The listing builds one solid part. Answer for the finished solid, in the listing's coordinates (mm). Face numbers are marked on the shaded views. A direction names the side the tool comes from. Coordinates: 2 decimals unless noted, no trailing zeros. Order: outer loops, then holes, each group sorted by start corner. A loop starts at its lowest first (then second) coordinate and runs counter-clockwise, first axis right, second up. Notation, with made-up numbers: (66.25, 51) -> (108.25, 51) arc R18 ccw to (108.25, 84) -> close; hole circle Ø10 at (-6, 8.25). An arc over 180 degrees is marked (long way). Return JSON: item names as keys, results as strings.
from build123d import *

# Parameters (mm, degrees)
SKETCH_1_W          = 40
SKETCH_1_H          = 30
EXTRUDE_1_DEPTH     = 5
SKETCH_2_R          = 1.5
CUT_EXTRUDE_1_DEPTH = 10
SKETCH_3_W          = 20
SKETCH_3_H          = 30
CUT_EXTRUDE_2_DEPTH = 1


with BuildPart() as part:
    # 草图1 → 凸台-拉伸1 (new body)
    with BuildSketch(Plane.XY):
        Rectangle(SKETCH_1_W, SKETCH_1_H)
    extrude(amount=EXTRUDE_1_DEPTH)

    # 草图2 → 切除-拉伸1 (cut)
    with BuildSketch(Plane(origin=(0, 0, 0), x_dir=(-1, 0, 0), z_dir=(0, 0, -1))):
        with Locations((14, 10)):
            Circle(SKETCH_2_R)
        with Locations((-14, 10)):
            Circle(SKETCH_2_R)
        with Locations((-14, -10)):
            Circle(SKETCH_2_R)
        with Locations((14, -10)):
            Circle(SKETCH_2_R)
    extrude(amount=-CUT_EXTRUDE_1_DEPTH, mode=Mode.SUBTRACT)

    # 草图3 → 切除-拉伸2 (cut)
    with BuildSketch(Plane.XY.offset(5)):
        Rectangle(SKETCH_3_W, SKETCH_3_H)
    extrude(amount=-CUT_EXTRUDE_2_DEPTH, mode=Mode.SUBTRACT)


solid = part.part
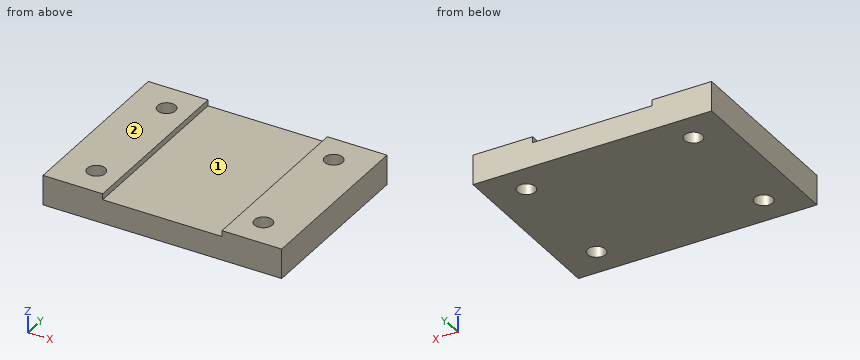
1. The part is cut by section A-A on y = 10. Give the vertices of the cut face in (x, z), and give its area (3 significant figures).
Answer block:
{"outline": "(-20, 0) -> (-15.5, 0) -> (-15.5, 5) -> (-20, 5) -> close; (-12.5, 0) -> (12.5, 0) -> (12.5, 5) -> (10, 5) -> (10, 4) -> (-10, 4) -> (-10, 5) -> (-12.5, 5) -> close; (15.5, 0) -> (20, 0) -> (20, 5) -> (15.5, 5) -> close", "area": "150 mm2"}
2. The part is cut by section B-B on x = -14. Give the vertices of the cut face in (y, z).
Answer block:
{"outline": "(-15, 0) -> (-11.5, 0) -> (-11.5, 5) -> (-15, 5) -> close; (-8.5, 0) -> (8.5, 0) -> (8.5, 5) -> (-8.5, 5) -> close; (11.5, 0) -> (15, 0) -> (15, 5) -> (11.5, 5) -> close"}
3. Consider line 1 (Y direction, x = -14, z = 3.65); line 2 (Y direction, x = -13, z = 2.45); line 3 (Z direction, x = -3, y = -8). Determine where each line is inside the solid, lowest interval first. Write a range as from..to.
Answer block:
{"line 1": "y = -15..-11.5, -8.5..8.5, 11.5..15", "line 2": "y = -15..-11.12, -8.88..8.88, 11.12..15", "line 3": "z = 0..4"}
4. The part is cut by section C-C on y = 5.5. Give the vertices of the cut face in (x, z).
Answer block:
{"outline": "(-20, 0) -> (20, 0) -> (20, 5) -> (10, 5) -> (10, 4) -> (-10, 4) -> (-10, 5) -> (-20, 5) -> close"}
5. For the marked faces 1 and 2, determine the directions among +Z, -Z, +X, -X, +Y, -Y from which every point of the face is accessible in a straight line to the end or side of a thin tool.
Answer block:
{"face 1": "+Z, +Y, -Y", "face 2": "+Z, +X, -X, +Y, -Y"}
6. Each of these flat-tipped pins is pushed along its axis until it touches: pin 1 Ø2.5 at (x, y) = (-14, 10) entering from +Z; pin 2 Ø5 at (x, y) = (-14, -10) entering from -Z; pin 3 Ø10 at (x, y) = (-2.5, -1.5) entering from +Z. Where does it stop, or does it pass through?
Answer block:
{"pin 1": "passes through", "pin 2": "stops at z = 0", "pin 3": "stops at z = 4"}
7. The part is cut by section D-D on x = 7. Give the vertices of the cut face in (y, z), and give its area (3 significant figures).
Answer block:
{"outline": "(-15, 0) -> (15, 0) -> (15, 4) -> (-15, 4) -> close", "area": "120 mm2"}
